Verification items for this drawing (mm, ordinates from the low corner). Give positions to 0.01 mm unless a question says otherwise; leave off trailing zeros. Loops run counter-clockwise (first coordinate to the right, second up) from the corner with the lowest first, then second, coordinate; pieces in that order, holes last. Notation, with made-up numbers: (15.25, 36.25) -> (25.25, 36.25) arc R27 cw to (25.25, 73.25) -> close; hole circle Ø6 at (-36.5, 47.25). An arc over 180 degrees is marked (long way). Write each question's results on one line, items separated by ' | '. Start each with the question number.
1) Sectioned sample at B-B on z = 27. Record the cut outline in (x, y) (3 decimals).
2) Sectioned sample at C-C on y = 8. Record the cut outline in (x, z) (3 decimals).
3) Depth check by flat-ended pin: pin 1 (1 mm diameter, centred on x = 1, z = 1, fed in from +Y) (3 decimals); pin 2 (1 mm diameter, centred on x = 1, z = 200.5, fed in from -Y) (3 decimals); pin 3 (1 mm diameter, centred on x = 1, z = 228, fed in from -Y) (3 decimals). Enter the tip coordinate at first touch or a pass-through.
4) Sectioned sample at A-A on x = 0.6. Record the cut outline in (y, z) (3 decimals), then the cut area to 3 significant figures.
5) Scan lines: line 1 (Z direction, x = 2.55, y = 34); line 2 (Y direction, x = 1.25, z = 148) (3 decimals); line 3 (Z direction, x = 2.45, y = 63) (3 decimals). Record each from-to range of solid material in increasing order. Write a range as from..to.
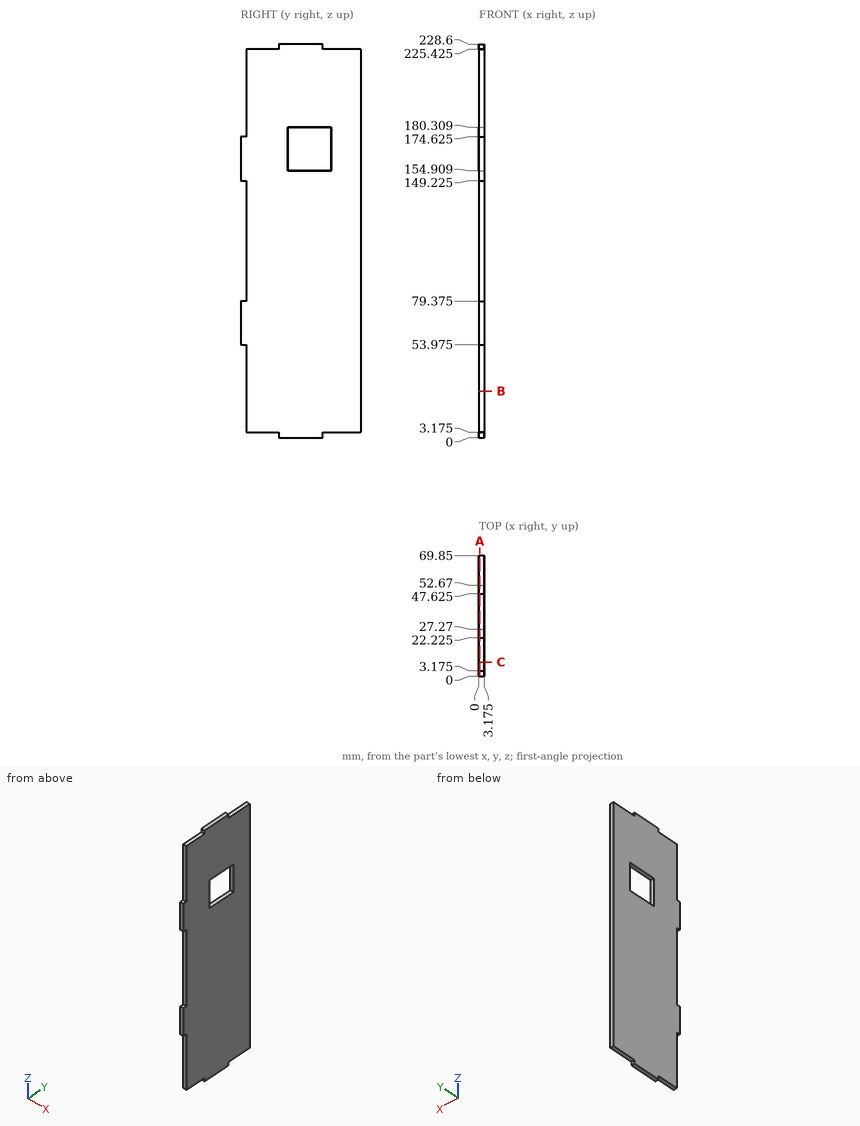
Result:
1) outline: (0, 3.175) -> (3.175, 3.175) -> (3.175, 69.85) -> (0, 69.85) -> close
2) outline: (0, 3.175) -> (3.175, 3.175) -> (3.175, 225.425) -> (0, 225.425) -> close
3) pin 1: y = 47.625 | pin 2: y = 3.175 | pin 3: y = 22.225
4) outline: (0, 53.975) -> (3.175, 53.975) -> (3.175, 3.175) -> (22.225, 3.175) -> (22.225, 0) -> (47.625, 0) -> (47.625, 3.175) -> (69.85, 3.175) -> (69.85, 225.425) -> (47.625, 225.425) -> (47.625, 228.6) -> (22.225, 228.6) -> (22.225, 225.425) -> (3.175, 225.425) -> (3.175, 174.625) -> (0, 174.625) -> (0, 149.225) -> (3.175, 149.225) -> (3.175, 79.375) -> (0, 79.375) -> close; hole (27.27, 154.909) -> (52.67, 154.909) -> (52.67, 180.309) -> (27.27, 180.309) -> close | area: 14,500 mm^2
5) line 1: 0..154.91, 180.31..228.6 | line 2: 3.175..69.85 | line 3: 3.175..225.425
